Part model, mm, in its own coordinate system. A direction names the side the tool comes from. Coordinates: 2 decimals unless noted, no trailing zeros. Loops run counter-clockwise (first coordinate to the right, second up) from the corner with the lowest first, then second, coordinate; pieces in that order, holes last. Notation, with made-up numbers: M 51.25,78 L 98.25,78 A27 ccw 98.25,109 Z; hole C 67,80 d6. An arc over 180 degrees is marked long. Answer as CSV lines item,"result". Start each with the question number.
Autodesk Inventor part; units mm, degrees
ref_plane "YZ Plane" through (0, 0, 0) normal (1, 0, 0) x (0, 1, 0)
ref_plane "XZ Plane" through (0, 0, 0) normal (0, 1, 0) x (-1, 0, 0)
ref_plane "XY Plane" through (0, 0, 0) normal (0, 0, 1) x (1, 0, 0)
sketch "Sketch1" plane through (0, 0, 0) normal (0, 1, 0) x (-1, 0, 0)
  line L0 (0, 0) -> (-90, 0)
  line L1 (-90, 0) -> (-90, -60)
  line L2 (-90, -60) -> (0, -60)
  line L3 (0, -60) -> (0, 0)
  dimension "d0" = 90
  dimension "d1" = 60
extrude "Extrusion1" add sketch "Sketch1" along normal blind 2
sketch "Sketch2" plane through (0, 2, 0) normal (0, 1, 0) x (1, 0, 0)
  line L0 (90, 0) -> (90, 60) construction
  line L1 (90, 60) -> (85, 60) construction
  line L2 (90, 60) -> (0, 60) construction
  line L3 (85, 60) -> (85, 0) construction
  line L4 (0, 0) -> (90, 0) construction
  line L5 (85, 30) -> (85, 35.5) construction
  line L6 (85, 35.5) -> (85, 30) construction
  line L7 (85, 30) -> (85, 24.5) construction
  line L8 (85, 24.5) -> (79, 24.5)
  line L9 (79, 24.5) -> (79, 23.5)
  line L10 (79, 23.5) -> (85, 23.5)
  line L11 (85, 23.5) -> (85, 24.5)
  line L12 (85, 35.5) -> (79, 35.5)
  line L13 (79, 35.5) -> (79, 36.5)
  line L14 (79, 36.5) -> (85, 36.5)
  line L15 (85, 36.5) -> (85, 35.5)
  dimension "d4" = 5
  dimension "d5" = 5.5
  dimension "d6" = 5.5
  dimension "d7" = 6
  dimension "d8" = 1
  dimension "d9" = 1
extrude "Extrusion2" cut sketch "Sketch2" against normal through all
sketch "Sketch3" plane through (0, 2, 0) normal (0, 1, 0) x (1, 0, 0)
  line L0 (85, 35.5) -> (79, 35.5) construction
  line L1 (85, 24.5) -> (79, 24.5) construction
  line L2 (79, 35.5) -> (79, 24.5) construction
  line L3 (79, 30) -> (72.5, 30) construction
  line L4 (72.5, 30) -> (72.5, 32.5) construction
  line L5 (72.5, 32.5) -> (67.5, 32.5) construction
  line L6 (67.5, 32.5) -> (67.5, 27.5) construction
  line L7 (67.5, 27.5) -> (72.5, 27.5) construction
  line L8 (72.5, 27.5) -> (72.5, 32.5) construction
  line L9 (67.5, 27.5) -> (70.5, 27.5) construction
  line L10 (67.5, 32.5) -> (70.5, 32.5) construction
  arc A0 (70.5, 27.5) -> (70.5, 32.5) centre (69.9375, 30) ccw
  line L11 (70.5, 32.5) -> (67.5, 32.5) construction
  line L12 (67.5, 32.5) -> (67.5, 27.5) construction
  line L13 (67.5, 32.5) -> (70.5, 32.5)
  line L14 (67.5, 32.5) -> (67.5, 27.5)
  line L15 (67.5, 27.5) -> (70.5, 27.5)
  point P0 (0, 0)
  dimension "d12" = 6.5
  dimension "d15" = 2.5
  dimension "d16" = 5
  dimension "d17" = 5
  dimension "d18" = 3
  dimension "d19" = 3
extrude "Extrusion3" cut sketch "Sketch3" against normal through all
sketch "Sketch5" plane through (0, 2, 0) normal (0, 1, 0) x (1, 0, 0)
  line L0 (85, 35.5) -> (85, 36.5) construction
  line L1 (85, 36.5) -> (67.5, 36.5) construction
  line L2 (67.5, 36.5) -> (67.5, 23.5) construction
  line L3 (67.5, 23.5) -> (85, 23.5) construction
  line L4 (85, 23.5) -> (85, 36.5) construction
  circle A0 centre (76.25, 30) radius 12.5 construction
  line L5 (76.25, 30) -> (85, 30) construction
  line L6 (85, 30) -> (85, 30.5) construction
  line L7 (85, 30.5) -> (76.25, 30.5)
  line L8 (76.25, 30.5) -> (76.25, 29.5)
  line L9 (76.25, 29.5) -> (85, 29.5)
  line L10 (85, 29.5) -> (85, 30.5)
  line L11 (76.25, 30) -> (71.875, 37.5777) construction
  line L12 (71.875, 37.5777) -> (71.442, 37.3277) construction
  line L13 (71.442, 37.3277) -> (75.817, 29.75)
  line L14 (75.817, 29.75) -> (76.683, 30.25)
  line L15 (76.683, 30.25) -> (72.308, 37.8277)
  line L16 (72.308, 37.8277) -> (71.442, 37.3277)
  line L17 (76.25, 30) -> (71.875, 22.4223) construction
  line L18 (71.875, 22.4223) -> (72.308, 22.1723) construction
  line L19 (72.308, 22.1723) -> (76.683, 29.75)
  line L20 (76.683, 29.75) -> (75.817, 30.25)
  line L21 (75.817, 30.25) -> (71.442, 22.6723)
  line L22 (71.442, 22.6723) -> (72.308, 22.1723)
  point P0 (0, 0)
  dimension "d32" = 13
  dimension "d33" = 25
  dimension "d34" = 0.5
  dimension "d35" = 1
  dimension "d38" = 360
extrude "Extrusion4" add sketch "Sketch5" along normal blind 10
sketch "Sketch6" plane through (0, 2, 0) normal (0, 1, 0) x (1, 0, 0)
  line L0 (85, 36.5) -> (85, 35.5) construction
  line L1 (85, 36.5) -> (67.5, 36.5) construction
  line L2 (67.5, 36.5) -> (67.5, 23.5) construction
  line L3 (67.5, 23.5) -> (85, 23.5) construction
  line L4 (85, 23.5) -> (85, 36.5) construction
  circle A0 centre (76.25, 30) radius 12.5
  circle A1 centre (76.25, 30) radius 13
  point P0 (0, 0)
  dimension "d42" = 13
  dimension "d43" = 25
  dimension "d44" = 26
extrude "Extrusion5" add sketch "Sketch6" along normal blind 6
sketch "Sketch7" plane through (0, 2, 0) normal (0, 1, 0) x (1, 0, 0)
  line L0 (90, 0) -> (90, 60) construction
  line L1 (90, 30) -> (90, 14) construction
  line L2 (90, 14) -> (0, 14) construction
  line L3 (0, 60) -> (0, 0) construction
  line L4 (90, 14) -> (85, 14) construction
  line L5 (85, 14) -> (11, 14) construction
  line L6 (11, 14) -> (11, 12.4) construction
  line L7 (11, 12.4) -> (85, 12.4) construction
  line L8 (85, 12.4) -> (85, 14) construction
  line L9 (85, 14) -> (85, 12.4)
  line L10 (85, 12.4) -> (80, 12.4)
  line L11 (85, 14) -> (80, 14)
  line L12 (80, 14) -> (80, 15.5)
  line L13 (80, 12.4) -> (80, 10.9)
  line L14 (11, 14) -> (16, 14)
  line L15 (16, 14) -> (16, 15.5)
  line L16 (16, 15.5) -> (9, 15.5)
  line L17 (11, 14) -> (11, 12.4)
  line L18 (11, 12.4) -> (16, 12.4)
  line L19 (16, 12.4) -> (16, 10.9)
  line L20 (16, 10.9) -> (9, 10.9)
  line L21 (9, 10.9) -> (9, 15.5)
  line L22 (80, 15.5) -> (86.5, 15.5)
  line L23 (80, 10.9) -> (86.5, 10.9)
  line L24 (86.5, 10.9) -> (86.5, 15.5)
  dimension "d47" = 16
  dimension "d48" = 5
  dimension "d49" = 74
  dimension "d50" = 1.6
  dimension "d51" = 5
  dimension "d52" = 5
  dimension "d53" = 1.5
  dimension "d55" = 1.5
  dimension "d57" = 5
  dimension "d58" = 1.5
  dimension "d59" = 7
  dimension "d60" = 5
  dimension "d61" = 1.5
  dimension "d62" = 6.5
  dimension "d63" = 6.5
extrude "Extrusion6" add sketch "Sketch7" along normal blind 4
sketch "Sketch8" plane through (0, 6, 0) normal (0, 1, 0) x (1, 0, 0)
  line L0 (80, 15.5) -> (80, 14)
  line L1 (80, 14) -> (80, 15.5)
  line L2 (86.5, 10.9) -> (86.5, 15.5)
  line L3 (80, 15.5) -> (86.5, 15.5)
  line L4 (86.5, 15.5) -> (86.5, 10.9)
  line L5 (80, 12.4) -> (80, 10.9)
  line L6 (86.5, 10.9) -> (80, 10.9)
  line L7 (80, 10.9) -> (80, 12.4)
  line L8 (85, 12.4) -> (80, 12.4)
  line L9 (80, 12.4) -> (85, 12.4)
  line L10 (85, 14) -> (85, 12.4)
  line L11 (85, 12.4) -> (85, 14)
  line L12 (80, 14) -> (85, 14)
  line L13 (85, 14) -> (80, 14)
  point P0 (0, 0)
extrude "Extrusion7" add sketch "Sketch8" along normal blind 4
sketch "Sketch10" plane through (0, 2, 0) normal (0, 1, 0) x (1, 0, 0)
  line L0 (90, 0) -> (90, 60) construction
  line L1 (90, 30) -> (50, 30) construction
  line L2 (50, 30) -> (50, 37.5) construction
  line L3 (50, 37.5) -> (10, 37.5)
  line L4 (10, 37.5) -> (10, 22.5)
  line L5 (10, 22.5) -> (50, 22.5)
  line L6 (50, 22.5) -> (50, 37.5)
  point P0 (0, 0)
  dimension "d82" = 40
  dimension "d83" = 7.5
  dimension "d84" = 40
  dimension "d85" = 15
extrude "Extrusion9" add sketch "Sketch10" along normal blind 15
sketch "Sketch11" plane through (10, 2, -22.5) normal (0, 0, 1) x (1, 0, 0)
  line L0 (0, 0) -> (0, 15) construction
  line L1 (0, 15) -> (20, 15) construction
  line L2 (40, 15) -> (0, 15) construction
  arc A0 (5, 15) -> (35, 15) centre (20, 15) ccw
  line L3 (5, 15) -> (35, 15)
  point P0 (-10, -2)
  dimension "d88" = 30
extrude "Extrusion10" cut sketch "Sketch11" against normal blind 15
sketch "Sketch15" plane through (0, 2, 0) normal (0, 1, 0) x (1, 0, 0)
  line L0 (90, 0) -> (90, 60) construction
  line L1 (90, 30) -> (90, 45) construction
  line L2 (90, 45) -> (90, 45) construction
  line L3 (90, 45) -> (68, 45) construction
  line L4 (68, 45) -> (68, 65) construction
  line L5 (68, 65) -> (90, 65) construction
  line L6 (90, 65) -> (90, 45) construction
  line L7 (68, 45) -> (68, 50)
  line L8 (68, 50) -> (66.5, 50)
  line L9 (66.5, 50) -> (66.5, 45)
  line L10 (66.5, 45) -> (66.5, 43.5)
  line L11 (68, 45) -> (73, 45)
  line L12 (73, 45) -> (73, 43.5)
  line L13 (73, 43.5) -> (66.5, 43.5)
  line L14 (90, 60) -> (0, 60)
  point P0 (0, 0)
  dimension "d99" = 15
  dimension "d100" = 0
  dimension "d101" = 22
  dimension "d102" = 20
  dimension "d103" = 5
  dimension "d104" = 1.5
  dimension "d105" = 5
  dimension "d106" = 1.5
extrude "Extrusion13" add sketch "Sketch15" along normal blind 5
sketch "Sketch17" plane through (0, 17, 0) normal (0, 1, 0) x (1, 0, 0)
  line L0 (50, 37.5) -> (45, 37.5)
  line L1 (45, 22.5) -> (30, 22.5)
  line L2 (50, 37.5) -> (45, 37.5)
  line L3 (45, 37.5) -> (45, 22.5)
  line L4 (45, 22.5) -> (50, 22.5)
  line L5 (50, 22.5) -> (50, 37.5)
  line L6 (15, 37.5) -> (30, 37.5)
  line L7 (30, 22.5) -> (10, 22.5)
  line L8 (15, 37.5) -> (10, 37.5)
  line L9 (10, 37.5) -> (10, 22.5)
  line L10 (10, 22.5) -> (15, 22.5)
  line L11 (15, 22.5) -> (15, 37.5)
  point P0 (0, 0)
extrude "Extrusion14" add sketch "Sketch17" along normal blind 5
sketch "Sketch18" plane through (0, 2, 0) normal (0, 1, 0) x (1, 0, 0)
  line L0 (90, 0) -> (90, 60) construction
  line L1 (90, 30) -> (90, 46) construction
  line L2 (90, 46) -> (0, 46) construction
  line L3 (66.5, 43.5) -> (66.5, 50) construction
  line L4 (66.5, 46) -> (65, 46) construction
  line L5 (65, 46) -> (13, 46) construction
  line L6 (13, 46) -> (13, 47.6) construction
  line L7 (13, 47.6) -> (65, 47.6) construction
  line L8 (65, 47.6) -> (65, 46) construction
  line L9 (65, 46) -> (60, 46)
  line L10 (60, 46) -> (60, 44.5)
  line L11 (60, 44.5) -> (66.5, 44.5)
  line L12 (65, 46) -> (65, 47.6)
  line L13 (65, 47.6) -> (60, 47.6)
  line L14 (60, 47.6) -> (60, 49.1)
  line L15 (60, 49.1) -> (66.5, 49.1)
  line L16 (66.5, 49.1) -> (66.5, 44.5)
  line L17 (13, 47.6) -> (13, 46)
  line L18 (13, 46) -> (18, 46)
  line L19 (18, 46) -> (18, 44.5)
  line L20 (18, 44.5) -> (11.5, 44.5)
  line L21 (13, 47.6) -> (18, 47.6)
  line L22 (18, 47.6) -> (18, 49.1)
  line L23 (18, 49.1) -> (11.5, 49.1)
  line L24 (11.5, 49.1) -> (11.5, 44.5)
  point P0 (0, 0)
  dimension "d115" = 16
  dimension "d116" = 1.5
  dimension "d117" = 52
  dimension "d118" = 1.6
  dimension "d119" = 5
  dimension "d120" = 1.5
  dimension "d121" = 5
  dimension "d122" = 1.5
  dimension "d123" = 5
  dimension "d124" = 1.5
  dimension "d125" = 6.5
  dimension "d126" = 1.5
extrude "Extrusion15" add sketch "Sketch18" along normal blind 5
sketch "Sketch19" plane through (0, 0, 0) normal (0, 0, 1) x (1, 0, 0)
  line L0 (90, 2) -> (0, 2)
  line L1 (90, 0) -> (0, 0)
  line L2 (0, 2) -> (90, 2)
  line L3 (90, 2) -> (90, 0)
  line L4 (90, 0) -> (0, 0)
  line L5 (0, 0) -> (0, 2)
extrude "Extrusion16" add sketch "Sketch19" along normal blind 1.5
sketch "Sketch20" plane through (90, 0, -60) normal (1, 0, 0) x (0, 0, -1)
  line L0 (0, 0) -> (0, 2)
  line L1 (0, 2) -> (-61.5, 2)
  line L2 (0, 0) -> (-61.5, 0)
  line L3 (-61.5, 0) -> (-61.5, 2)
  line L4 (-61.5, 2) -> (0, 2)
  line L5 (0, 2) -> (0, 0)
  point P0 (-60, 0)
extrude "Extrusion17" add sketch "Sketch20" along normal blind 1.25
sketch "Sketch21" plane through (0, 0, -60) normal (0, 0, -1) x (-1, 0, 0)
  line L0 (0, 0) -> (-91.25, 0)
  line L1 (-91.25, 0) -> (-91.25, 2)
  line L2 (-91.25, 2) -> (0, 2)
  line L3 (0, 2) -> (0, 0)
extrude "Extrusion18" add sketch "Sketch21" along normal blind 7
sketch "Sketch22" plane through (0, 2, 0) normal (0, 1, 0) x (1, 0, 0)
  line L0 (85, 30.5) -> (85, 29.5) construction
  line L1 (91.25, -1.5) -> (91.25, 67) construction
  line L2 (91.25, 30) -> (89.25, 30) construction
  line L3 (89.25, 30) -> (87.75, 30) construction
  line L4 (87.75, 30) -> (87.75, 18.5) construction
  line L5 (87.75, 18.5) -> (50.75, 18.5) construction
  line L6 (50.75, 18.5) -> (50.75, 41.5) construction
  line L7 (50.75, 41.5) -> (87.75, 41.5) construction
  line L8 (87.75, 41.5) -> (87.75, 18.5) construction
  point P0 (0, 0)
  dimension "d135" = 2
  dimension "d136" = 1.5
  dimension "d137" = 11.5
  dimension "d138" = 37
  dimension "d139" = 23
properties part number "base"
Q1. Tool access for faces 5 (the face through (70, 4, -43.5)), 6 (the face through (82, 1, -35.5)), 7 (the face through (83, 6, -12.4)), 8 (the face through (70, 4, -45)), 9 (the face through (63, 4, -44.5)): list every direction of +Z, -Z, +X, -X, +Y, -Y with a clear straight run to the whole face (end or side of a thin tool).
Q2. Slice it at B-B, the plane x = 46. Write the cut outline in (y, z), and give its area (3 significant figures).
Q3. Wall check: L1, parallel to X at y = 19, z = -27; L2, parallel to Z at x = 76.25, y = 3.5; L3, parallel to X at y = 4.95, z = -30. Give the ranges that are in metal, low to high.
Q4. Flat gauge pins, fed straight in: P1, Ø12, axis at x = 57, z = -39.5, coming from the +Y side; P2, Ø1, axis at x = 73.5, z = -11, coming from the +Y side; P3, Ø5.5, axis at x = 61.5, y = 4, coming from the -Z side; P4, Ø6, axis at y = 7, z = -14.5, coming from the -X side. Where does each tip first touch, or does it go through?
Q5. Slice it at A-A, the plane y = 18.25. Write the cut outline in (x, z), and give its area (3 significant figures).
Q6. Slice it at C-C, the plane y = 4.25. State how many separate pieces and enclosed holes the cut face has, and give its area (3 significant figures).
Q7. Two-plate mould, pull along Z, no slides. Class faces 1 (the face through (45, 1, 1.5)), 2 (the face through (91.25, 1, -32)), 3 (the face through (74.453, 6.93, -34.113)), 4 (the face through (63, 4, -49.1)): +Z half, -Z half, draft (parallel to the pull), parting line (faces both ways), or undercut.
Q8. Slice it at D-D, the plane z = -55. Write the cut outline in (x, y), and give its area (4 significant figures).
Solved:
1,face 5,"+X, -X, +Y"
1,face 6,"+Y, -Y"
1,face 7,"+Y"
1,face 8,"-Z, +X, +Y"
1,face 9,"-X, +Y"
2,outline,"M 0,-67 L 2,-67 L 2,-37.5 L 22,-37.5 L 22,-22.5 L 2,-22.5 L 2,1.5 L 0,1.5 Z"
2,area,"437 mm2"
3,L1,"x = 10 to 15, 45 to 50"
3,L2,"z = -43 to -42.5, -31 to -29, -17.5 to -17"
3,L3,"x = 10 to 21.07, 38.93 to 50, 63.25 to 63.75, 75.67 to 85, 88.75 to 89.25"
4,P1,"stops at y = 7"
4,P2,"stops at y = 2"
4,P3,"stops at z = -67"
4,P4,"stops at x = 9"
5,outline,"M 10,-37.5 L 15,-37.5 L 15,-22.5 L 10,-22.5 Z; M 45,-37.5 L 50,-37.5 L 50,-22.5 L 45,-22.5 Z"
5,area,"150 mm2"
6,separate pieces,"8"
6,enclosed holes,"1"
6,area,"536 mm2"
7,face 1,"+Z half"
7,face 2,"draft"
7,face 3,"undercut"
7,face 4,"-Z half"
8,outline,"M 0,0 L 91.25,0 L 91.25,2 L 0,2 Z"
8,area,"182.5 mm2"
